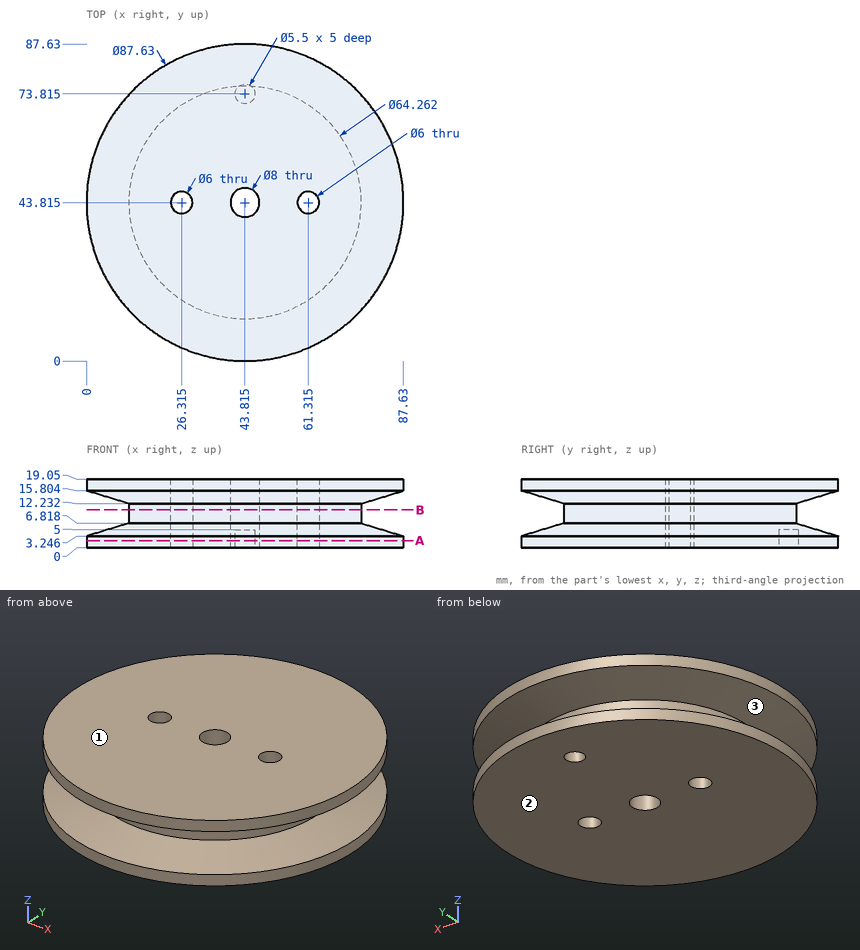
Study the drawing (mm; zero at the part's minimum x, y, z) and answer. Coordinates: 2 decimals unless noted, no trailing zeros. Loops run counter-clockwise (first coordinate to the right, second up) from the corner with the lowest first, then second, coordinate; pieces in that order, holes last. Notation, with made-up numbers: M 18,47.5 L 49,47.5 A20 cw 49,71.5 Z; hole C 56,51 d11. An arc over 180 degrees is marked long. Answer in a Markdown table with one row per item. Add a question column.
1. Find section B-B, the plane z = 10.5. Write down the section's boundary in (x, y) (1 decimal), then the cut area to 3 significant figures.
2. Find section A-A, the plane z = 2. State how many separate pieces and enclosed holes the cut face has, then the cut area to 3 significant figures.
3. Consider L1, parallel to X at y = 43.5, z = 2; L2, parallel to Z at x = 31, y = 82; L3, parallel to Z at x = 5, y = 62.5. Determine where each line is inside the solid, lowest interval first.
4. The mould has two halves that part along Z. Classify the marked faces 1, 2 and 3: pulls with the +Z half, pulls with the -Z half, needs draft (parallel to the pull), parting line crosses it, or undercut.
5. Flat-ended cylindrical pins translate along their axes: P1, Ø12, axis at x = 56.5, y = 38.5, coming from the -Z side; P2, Ø5, axis at x = 43.815, y = 73.815, coming from the -Z side; P3, Ø1.5, axis at x = 21.5, z = 3.5, coming from the -Y side; P4, Ø10, axis at y = 35, z = 2, coming from the -X side. Find the tip coordinate at first contact, or state that the pin passes through.
Reported:
| question | item | result |
|---|---|---|
| 1 | outline | C 43.8,43.8 d64.3; hole C 26.3,43.8 d6; hole C 43.8,43.8 d8; hole C 61.3,43.8 d6 |
| 1 | area | 3,140 mm^2 |
| 2 | separate pieces | 1 |
| 2 | enclosed holes | 4 |
| 2 | area | 5,900 mm^2 |
| 3 | L1 | x = 0 to 23.33, 29.3 to 39.83, 47.8 to 58.33, 64.3 to 87.63 |
| 3 | L2 | z = 0 to 4.33, 14.72 to 19.05 |
| 3 | L3 | z = 0 to 3.47, 15.58 to 19.05 |
| 4 | face 1 | pulls with the +Z half |
| 4 | face 2 | pulls with the -Z half |
| 4 | face 3 | undercut |
| 5 | P1 | stops at z = 0 |
| 5 | P2 | stops at z = 5 |
| 5 | P3 | stops at y = 5.7 |
| 5 | P4 | stops at x = 0.17 |
